from build123d import *

# Parameters (mm, degrees)
SKETCH133_W             = 52.5
SKETCH133_H             = 56.5
SKETCH133_W_2           = 42.5
SKETCH133_H_2           = 47
PAD067_DEPTH            = 37
SKETCH131_W             = 23
SKETCH131_H             = 33
POCKET057_DEPTH         = 5
SKETCH135_W             = 52.5
SKETCH135_H             = 56.5
SKETCH135_W_2           = 47
SKETCH135_H_2           = 52
PAD066_DEPTH            = 20
BODY037_PLACEMENT_ANGLE = 90


with BuildPart() as part:
    # Sketch133 → Pad067 (new body)
    with BuildSketch(Plane.XY):
        with Locations((0, -26)):
            Rectangle(SKETCH133_W, SKETCH133_H)
        with Locations((0, -25.75)):
            Rectangle(SKETCH133_W_2, SKETCH133_H_2, mode=Mode.SUBTRACT)
    extrude(amount=PAD067_DEPTH)

    # Sketch131 (on Face1 of Pad067) → Pocket057 (cut)
    with BuildSketch(Plane(origin=(0, 2.25, 0), x_dir=(-1, 0, 0), z_dir=(0, 1, 0))):
        with Locations((0, 20.5)):
            Rectangle(SKETCH131_W, SKETCH131_H)
    extrude(amount=-POCKET057_DEPTH, mode=Mode.SUBTRACT)

    # Sketch135 (on Face2 of Pocket057) → Pad066 (join)
    with BuildSketch(Plane(origin=(0, 0, 0), x_dir=(1, 0, 0), z_dir=(0, 0, -1))):
        with Locations((0, 26)):
            Rectangle(SKETCH135_W, SKETCH135_H)
        with Locations((0, 26)):
            Rectangle(SKETCH135_W_2, SKETCH135_H_2, mode=Mode.SUBTRACT)
    extrude(amount=PAD066_DEPTH)


with BuildPart() as part_1:
    # Body037 placement: moved
    add(part.part.moved(Location((0, 0, 135))).rotate(Axis((0, 0, 135), (0, 0, 1)), BODY037_PLACEMENT_ANGLE))


solid = part_1.part
Read the model definition and answer for the solid it produces. Units are mm, in the model's axes. A direction names the side the tool comes from. Coordinates: 2 decimals unless noted, no trailing zeros. Loops run counter-clockwise (first coordinate to the right, second up) from the corner with the lowest first, then second, coordinate; pieces in that order, holes last. Notation, with made-up numbers: (-1, -39.75) -> (58, -39.75) arc R13 cw to (58, -27.75) -> close; hole circle Ø3 at (68, 82). An arc over 180 degrees is marked (long way). Answer in a Markdown table with one row per item.
Item 1: A cutting plane is placed at C-C on z = 122.5. Determine the outline of the cut face in (x, y).
Returned:
| item | result |
|---|---|
| outline | (-2.25, -26.25) -> (54.25, -26.25) -> (54.25, 26.25) -> (-2.25, 26.25) -> close; hole (0, -23.5) -> (52, -23.5) -> (52, 23.5) -> (0, 23.5) -> close |
Item 2: Each of these flat-tipped pins is pushed along its axis until it touches: P1, Ø5, axis at x = -1, y = -0.5, coming from the +Z side; P2, Ø8, axis at x = 9.5, y = 4, coming from the +Z side; P3, Ø12, axis at x = 45.5, y = 17, coming from the -Z side. Where does it stop, or does it pass through?
Returned:
| item | result |
|---|---|
| P1 | stops at z = 139 |
| P2 | passes through |
| P3 | stops at z = 135 |
Item 3: A cutting plane is placed at A-A on x = 9. Determine the outline of the cut face in (y, z), plus the area to 3 significant figures.
Returned:
| item | result |
|---|---|
| outline | (-26.25, 115) -> (-23.5, 115) -> (-23.5, 135) -> (-21.25, 135) -> (-21.25, 172) -> (-26.25, 172) -> close; (21.25, 135) -> (23.5, 135) -> (23.5, 115) -> (26.25, 115) -> (26.25, 172) -> (21.25, 172) -> close |
| area | 480 mm^2 |
Item 4: A cutting plane is placed at B-B on y = -2. Determine the outline of the cut face in (x, z).
Returned:
| item | result |
|---|---|
| outline | (-2.25, 115) -> (0, 115) -> (0, 135) -> (2.25, 135) -> (2.25, 139) -> (-2.25, 139) -> close; (49.25, 135) -> (52, 135) -> (52, 115) -> (54.25, 115) -> (54.25, 172) -> (49.25, 172) -> close |
Item 5: A cutting plane is placed at D-D on z = 147.5. Determine the outline of the cut face in (x, y).
Returned:
| item | result |
|---|---|
| outline | (-2.25, -26.25) -> (54.25, -26.25) -> (54.25, 26.25) -> (-2.25, 26.25) -> (-2.25, 11.5) -> (2.25, 11.5) -> (2.25, 21.25) -> (49.25, 21.25) -> (49.25, -21.25) -> (2.25, -21.25) -> (2.25, -11.5) -> (-2.25, -11.5) -> close |
Item 6: For a pull along Y with two mould halves and no side action, classify faces 1 (the flat face through (26, -25, 115)), 2 (the flat face through (26, 23.5, 125)), 3 (the flat face through (26, -23, 135)), 4 (the flat face through (26, 26.25, 144)) as released by +Y, released by -Y, zero draft, split by the parting line, or undercut.
Returned:
| item | result |
|---|---|
| face 1 | zero draft |
| face 2 | undercut |
| face 3 | undercut |
| face 4 | released by +Y |
Item 7: Straight lines are drawn through the part: line 1 along X through (y, z) = (18, 169); line 2 along Y through (x, z) = (30.5, 127.5); line 3 along X through (y, z) = (1, 129.5). For each, find the intervals that lie inside material, in ascending order. Write a range as [from, to].
Returned:
| item | result |
|---|---|
| line 1 | x = [-2.25, 2.25], [49.25, 54.25] |
| line 2 | y = [-26.25, -23.5], [23.5, 26.25] |
| line 3 | x = [-2.25, 0], [52, 54.25] |
Item 8: For faces 5 (the flat face through (30, -22, 172)), 6 (the flat face through (26, -23.5, 125)), 7 (the flat face through (26, 21.25, 153)), 8 (the flat face through (54.25, 0, 144)), 9 (the flat face through (0, 0, 139)), determine the directions among +Z, -Z, +X, -X, +Y, -Y from which every point of the face is accessible in a straight line to the end or side of a thin tool.
Returned:
| item | result |
|---|---|
| face 5 | +Z, +X, -X, +Y, -Y |
| face 6 | -Z |
| face 7 | +Z, -Z |
| face 8 | +Z, -Z, +X, +Y, -Y |
| face 9 | +Z, -X |
